Work out the finished part from the listing and answer in its coordinate system (mm). Coordinates: 2 decimals unless noted, no trailing zeros. Order: outer loops, then holes, each group sorted by start corner. A loop starts at its lowest first (then second) coordinate and runs counter-clockwise, first axis right, second up.
1. Flat-ended cylindrical pins translate along their axes: pin 1 Ø1.5 at (y, z) = (-31.5, 3) entering from +X; pin 2 Ø1.9 at (x, y) = (-0.5, -29.5) entering from +Z; pin 3 Ø0.7 at (x, y) = (0, -30) entering from +Z. Find the tip coordinate at first contact, or state that the pin passes through.
2. Find the intervals of material crossed by probe 1 along Y at (x, z) = (0, 15.3); probe 2 along Y at (x, z) = (31, 3.25); probe 3 along Y at (x, z) = (0, 18.15), in increasing order.
3. The part is cut by section B-B, the plane z = 9.25. Give the vertices of the cut face in (x, y), then the cut area to 3 significant figures.
4. The part is cut by section D-D, the plane x = 0. Give the vertices of the cut face in (y, z).
5. The part is cut by section A-A, the plane x = -32.5. Give the vertices of the cut face in (y, z), then the cut area to 3 significant figures.
6. The part is cut by section C-C, the plane y = -29.5. Give the vertices of the cut face in (x, z), then the cut area to 3 significant figures.
```python
from build123d import *

# Parameters (mm, degrees)
F0_W     = 96
F0_H     = 72
F1_DEPTH = 19
F2_R     = 5
F3_R     = 0.5
F4_R     = 2
F5_DEPTH = 10
F6_R     = 1.1
F7_DEPTH = 5
F6_R_2   = 3.1
F8_DEPTH = 1.2


with BuildPart() as f1:
    # F0 (on Top) → F1 (new body)
    with BuildSketch(Plane.XY):
        Rectangle(F0_W, F0_H)
    extrude(amount=F1_DEPTH)

    # F2
    f2_edges = [f1.edges().sort_by_distance(p)[0] for p in [
        (48, 0, 19),
        (48, 0, 0),
        (-48, 0, 19),
        (-48, 0, 0),
    ]]
    fillet(f2_edges, radius=F2_R)

    # F3
    f3_edges = [f1.edges().sort_by_distance(p)[0] for p in [
        (-48, -36, 9.5),
        (-46.535534, -36, 1.464466),
        (-46.535534, -36, 17.535534),
        (0, -36, 0),
        (0, -36, 19),
        (46.535534, -36, 1.464466),
        (46.535534, -36, 17.535534),
        (48, -36, 9.5),
        (48, 36, 9.5),
        (46.535534, 36, 1.464466),
        (46.535534, 36, 17.535534),
        (0, 36, 0),
        (0, 36, 19),
        (-46.535534, 36, 1.464466),
        (-46.535534, 36, 17.535534),
        (-48, 36, 9.5),
    ]]
    fillet(f3_edges, radius=F3_R)

    # F4 (on face) → F5 (join)
    with BuildSketch(Plane.XZ.offset(36)):
        with Locations((-9.3, 3.75)):
            Circle(F4_R)
    extrude(amount=F5_DEPTH)

    # F6 (on face) → F7 (cut)
    with BuildSketch(Plane.XY.offset(19)):
        with Locations((0, -29.5)):
            Circle(F6_R)
    extrude(amount=-F7_DEPTH, mode=Mode.SUBTRACT)

    # F6 (on face) → F8 (cut)
    with BuildSketch(Plane.XY.offset(19)):
        with Locations((0, -29.5)):
            Circle(F6_R_2)
        with Locations((0, -29.5)):
            Circle(F6_R, mode=Mode.SUBTRACT)
    extrude(amount=-F8_DEPTH, mode=Mode.SUBTRACT)


solid = f1.part
```
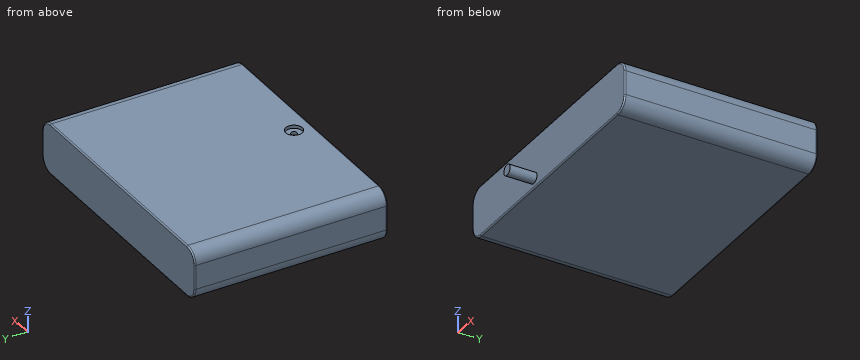
Geometry says:
1. pin 1: stops at x = 47.84
1. pin 2: stops at z = 17.8
1. pin 3: stops at z = 14
2. probe 1: y = -36 to -30.6, -28.4 to 36
2. probe 2: y = -36 to 36
2. probe 3: y = -36 to -32.6, -26.4 to 36
3. outline: (-48, -35.5) arc R0.5 ccw to (-47.5, -36) - (47.5, -36) arc R0.5 ccw to (48, -35.5) - (48, 35.5) arc R0.5 ccw to (47.5, 36) - (-47.5, 36) arc R0.5 ccw to (-48, 35.5) - close
3. area: 6,910 mm2
4. outline: (-36, 0.5) arc R0.5 ccw to (-35.5, 0) - (35.5, 0) arc R0.5 ccw to (36, 0.5) - (36, 18.5) arc R0.5 ccw to (35.5, 19) - (-26.4, 19) - (-26.4, 17.8) - (-28.4, 17.8) - (-28.4, 14) - (-30.6, 14) - (-30.6, 17.8) - (-32.6, 17.8) - (-32.6, 19) - (-35.5, 19) arc R0.5 ccw to (-36, 18.5) - close
5. outline: (-36, 0.5) arc R0.5 ccw to (-35.5, 0) - (35.5, 0) arc R0.5 ccw to (36, 0.5) - (36, 18.5) arc R0.5 ccw to (35.5, 19) - (-35.5, 19) arc R0.5 ccw to (-36, 18.5) - close
5. area: 1,370 mm2
6. outline: (-48, 5) arc R5 ccw to (-43, 0) - (43, 0) arc R5 ccw to (48, 5) - (48, 14) arc R5 ccw to (43, 19) - (3.1, 19) - (3.1, 17.8) - (1.1, 17.8) - (1.1, 14) - (-1.1, 14) - (-1.1, 17.8) - (-3.1, 17.8) - (-3.1, 19) - (-43, 19) arc R5 ccw to (-48, 14) - close
6. area: 1,790 mm2
